Design review of the part built by this model. Coordinates are the model's own, in mm. Give positions to 0.01 mm unless a question says otherwise; leave off trailing zeros. Order: outer loops, then holes, each group sorted by start corner. A loop starts at its lowest first (then second) coordinate and runs counter-clockwise, first axis right, second up.
Autodesk Inventor part; units mm, degrees
ref_plane "YZ Plane" through (0, 0, 0) normal (1, 0, 0) x (0, 1, 0)
ref_plane "XZ Plane" through (0, 0, 0) normal (0, 1, 0) x (-1, 0, 0)
ref_plane "XY Plane" through (0, 0, 0) normal (0, 0, 1) x (1, 0, 0)
sketch "Sketch1" plane through (0, 0, 0) normal (0, 0, 1) x (1, 0, 0)
  line L0 (0, 0) -> (0, 5)
  line L1 (0, 0) -> (12.7, 0)
  line L2 (12.7, 0) -> (12.7, 2.5)
  line L3 (12.7, 2.5) -> (0, 2.5)
  line L4 (0, 2.5) -> (0, 0)
  circle A0 centre (8.6603, 0) radius 10
  line L5 (-11, 1) -> (-1, 1)
  line L6 (-1, 1) -> (-1, -1)
  line L7 (-1, -1) -> (-11, -1)
  line L8 (-11, -1) -> (-11, 1)
  line L9 (0, 0) -> (-1, 0)
  line L10 (12.7, 2.5) -> (12.2, 2.5)
  line L11 (12.2, 2.5) -> (12.2, 2)
  line L12 (12.2, 2) -> (12.7, 2)
  line L13 (12.7, 2) -> (12.7, 2.5)
  circle A1 centre (12.7, 0) radius 2.5
  line L14 (12.7, 0) -> (15.2, 0)
  point P0 (-1.2896, 1)
  dimension "d3" = 20
  dimension "d0" = 5
  dimension "d1" = 12.7
  dimension "d2" = 2.5
  dimension "d4" = 1
  dimension "d5" = 1
  dimension "d6" = 1
  dimension "d7" = 10
  dimension "d8" = 0.5
  dimension "d9" = 0.5
revolve "Revolution1" add sketch "Sketch1" angle 360 about axis through (0, 0, 0) along (1, 0, 0) contours L9 L6 L5 A0 L0 | L0 L3 L11 A1 L1 | A1 L11 L12 L2 L1 | L2 A1 L14
equation "\"d6\" = d4"
properties part number "M5 x 12.7 Rivet"
1. Take a section at A-A (z = 0). State the section outline as (x, y) points.
Recorded:
outline: (-1.29, -1) arc R10 ccw to (0, -5) - (0, -2.5) - (12.2, -2.5) - (12.2, -2) - (12.7, -2) - (12.7, -2.5) arc R2.5 ccw to (12.7, 2.5) - (12.7, 2) - (12.2, 2) - (12.2, 2.5) - (0, 2.5) - (0, 5) arc R10 ccw to (-1.29, 1) - (-1, 1) - (-1, -1) - close
2. Draft analysis for pull direction X (two halves, no side actions). For faces 1 (the face through (-1, 0, 0)), 2 (the face through (6.01, -0.54, 2.44)), 3 (the face through (12.454, -0.434, -1.952)), 4 (the face through (0, 2, -2)), state which applies: pulls with the +X half, pulls with the -X half, needs draft (parallel to the pull), parting line crosses it, or undercut.
Recorded:
face 1: pulls with the -X half
face 2: needs draft
face 3: undercut
face 4: pulls with the +X half
3. For line 1 along Z through (x, y) = (8.75, 0); line 2 along Z through (x, y) = (10.5, -2); line 3 along Y through (x, z) = (5.5, 0.5), list the stretches that pass through material, from the lowest coordinate up.
Recorded:
line 1: z = -2.5 to 2.5
line 2: z = -1.5 to 1.5
line 3: y = -2.45 to 2.45
4. Take a section at C-C (y = 2.25). State the section outline as (x, z) points.
Recorded:
outline: (0, -4.47) - (0, -1.09) - (12.2, -1.09) - (12.2, 1.09) - (0, 1.09) - (0, 4.47) arc R9.74 ccw to start; (12.7, -1.09) arc R1.09 ccw to (12.7, 1.09) - close
5. Take a section at D-D (x = 11). State the section outline as (y, z) points.
Recorded:
outline: circle Ø5 at (0, 0)
6. For pin 1 (3 mm diameter, centred on x = 11, y = -3.5, fed in from +Z); pin 2 (6 mm diameter, centred on y = -3.5, z = 2, fed in from -X); pin 3 (1.5 mm diameter, centred on x = 7, y = 2, fed in from -Z), all flat-tipped, find the tip position at first contact; note any pin that passes through.
Recorded:
pin 1: stops at z = 1.5
pin 2: stops at x = -1.29
pin 3: stops at z = -2.17
